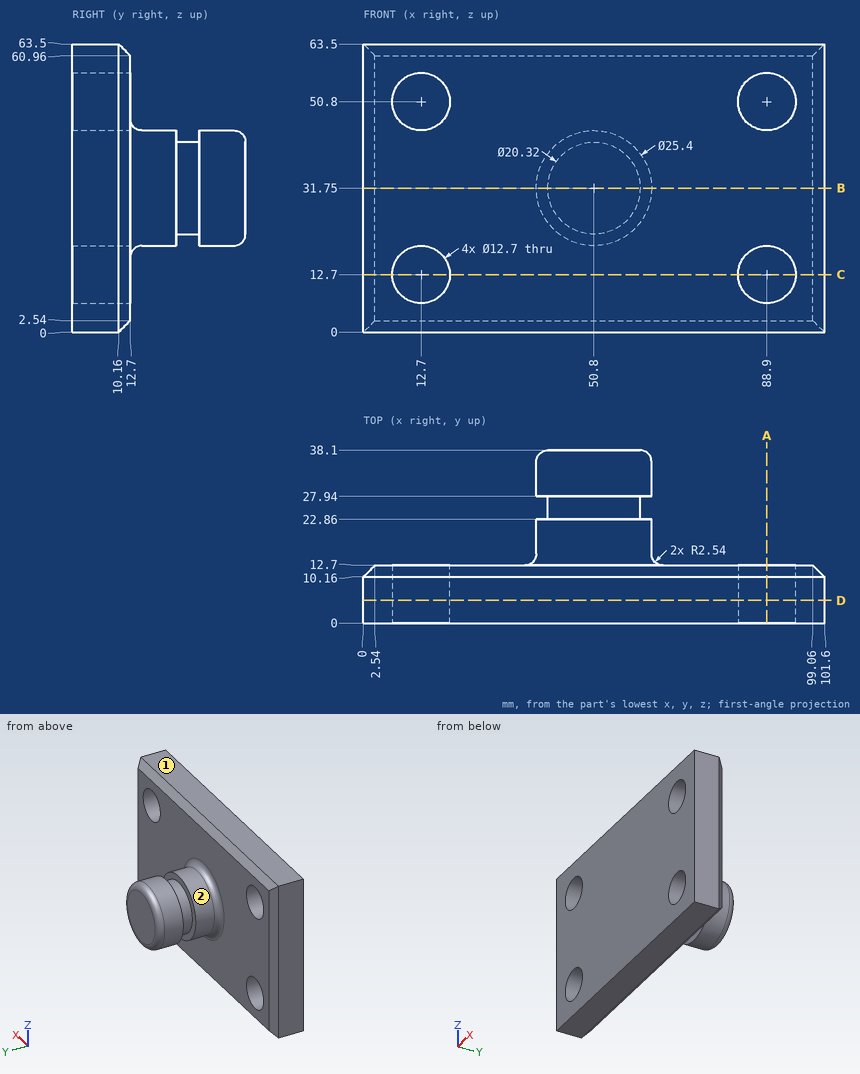
Design review of the part shown in the three views and the two pictorial views. Dimensions are in mm from the part's minimum x, y and z. A direction names the side the tool comes from. Give positions to 0.01 mm unless a question says otherwise; leave off trailing zeros. Write each loop counter-clockwise with the first axis right and the second up, starting at its lowest first coordinate (ties: lowest second). Pieces come first, ordered by that corner, then holes.
Item 1: Take a section at B-B (z = 31.75). Give the boundary of the cut face in (x, y).
Item 2: Wall thickness on probe 1 along Z at (x, y) = (12.7, 8.75); probe 2 along Z at (x, y) = (9, 6.5); probe 3 along Y at (x, z) = (63.5, 14): over which ranges is each line inside the solid? List them lowest first.
Item 3: Machinability: for the marked faces 1 and 2, which of the approach directions +Z, -Z, +X, -X, +Y, -Y give a long, thin tool a straight path to every point of the face, cutting with its end or side? Answer none if there is none.
Item 4: Take a section at C-C (z = 12.7). Give the boundary of the cut face in (x, y).
Item 5: Take a section at D-D (y = 5). Give the boundary of the cut face in (x, z), and give its area (3 significant figures).
Item 6: Take a section at A-A (x = 88.9). Give the boundary of the cut face in (y, z).
Item 7: Insertion check: P1, Ø12, axis at y = 22.5, z = 23.5, coming from the -X side; P2, Ø10, axis at x = 33.5, z = 42, coming from the +Y side; P3, Ø7.5, axis at x = 88.9, z = 12.7, coming from the +Y side. Each pin has a flat end and moves straight along its axis. Give the tip position at first contact, or say it passes through.
Established:
1. outline: (0, 0) - (101.6, 0) - (101.6, 10.16) - (99.06, 12.7) - (66.04, 12.7) arc R2.54 cw to (63.5, 15.24) - (63.5, 22.86) - (60.96, 22.86) - (60.96, 27.94) - (63.5, 27.94) - (63.5, 35.56) arc R2.54 ccw to (60.96, 38.1) - (40.64, 38.1) arc R2.54 ccw to (38.1, 35.56) - (38.1, 27.94) - (40.64, 27.94) - (40.64, 22.86) - (38.1, 22.86) - (38.1, 15.24) arc R2.54 cw to (35.56, 12.7) - (2.54, 12.7) - (0, 10.16) - close
2. probe 1: z = 0 to 6.35, 19.05 to 44.45, 57.15 to 63.5
2. probe 2: z = 0 to 7.54, 17.86 to 45.64, 55.96 to 63.5
2. probe 3: y = 0 to 12.7
3. face 1: +Z, +X, -X, +Y, -Y
3. face 2: +Y
4. outline: (0, 0) - (6.35, 0) - (6.35, 12.7) - (2.54, 12.7) - (0, 10.16) - close; (19.05, 0) - (82.55, 0) - (82.55, 12.7) - (19.05, 12.7) - close; (95.25, 0) - (101.6, 0) - (101.6, 10.16) - (99.06, 12.7) - (95.25, 12.7) - close
5. outline: (0, 0) - (101.6, 0) - (101.6, 63.5) - (0, 63.5) - close; hole circle Ø12.7 at (12.7, 12.7); hole circle Ø12.7 at (12.7, 50.8); hole circle Ø12.7 at (88.9, 12.7); hole circle Ø12.7 at (88.9, 50.8)
5. area: 5,940 mm2
6. outline: (0, 0) - (10.16, 0) - (12.7, 2.54) - (12.7, 6.35) - (0, 6.35) - close; (0, 19.05) - (12.7, 19.05) - (12.7, 44.45) - (0, 44.45) - close; (0, 57.15) - (12.7, 57.15) - (12.7, 60.96) - (10.16, 63.5) - (0, 63.5) - close
7. P1: stops at x = 38.3
7. P2: stops at y = 12.7
7. P3: passes through
